from build123d import *

# Parameters (mm, degrees)
CROQUIS1_W                                           = 50
CROQUIS1_H                                           = 50
CROQUIS1_R                                           = 2
SALIENTE_EXTRUIR2_DEPTH                              = 100
CROQUIS4_W                                           = 3.2
CROQUIS4_H                                           = 40
SALIENTE_EXTRUIR5_DEPTH                              = 10.2
CROQUIS8_R                                           = 4
CORTAR_EXTRUIR3_DEPTH                                = 87.4
CORTAR_EXTRUIR2_START                                = -50
CROQUIS7_R                                           = 2
CORTAR_EXTRUIR2_DEPTH                                = 50
REFRENTADO_PARA_TORNILLO_TAP_N_CON_CABEZ_D           = 4.5
REFRENTADO_PARA_TORNILLO_TAP_N_CON_CABEZ_CSINK_D     = 8.96
REFRENTADO_PARA_TORNILLO_TAP_N_CON_CABEZ_CSINK_ANGLE = 90
SALIENTE_EXTRUIR6_DEPTH                              = 1.95
SALIENTE_EXTRUIR7_START                              = -4.5
SALIENTE_EXTRUIR7_DEPTH                              = 1.95
CORTAR_EXTRUIR4_DEPTH                                = 15.4


with BuildPart() as part:
    # Croquis1 → Saliente-Extruir2 (new body)
    with BuildSketch(Plane.XY):
        Rectangle(CROQUIS1_W, CROQUIS1_H)
        Circle(CROQUIS1_R, mode=Mode.SUBTRACT)
    extrude(amount=SALIENTE_EXTRUIR2_DEPTH)

    # Croquis2 → Cortar-Revolución1 (revolve, cut)
    with BuildSketch(Plane(origin=(0, 0, 0), x_dir=(0, 0, -1), z_dir=(1, 0, 0))):
        Polygon((-100, 15.2), (-100, 0), (-89.8, 0), (-89.8, 10), (-97.8, 15.2), align=None)
    revolve(axis=Axis((0, 0, 100), (0, 0, -1)), mode=Mode.SUBTRACT)

    # Croquis4 → Saliente-Extruir5 (add)
    with BuildSketch(Plane.XY.offset(100)):
        with Locations((-6.6, 0)):
            Rectangle(CROQUIS4_W, CROQUIS4_H)
        with Locations((6.6, 0)):
            Rectangle(CROQUIS4_W, CROQUIS4_H)
    extrude(amount=-SALIENTE_EXTRUIR5_DEPTH)

    # Croquis8 → Cortar-Extruir3 (cut)
    with BuildSketch(Plane.XY.offset(89.8)):
        Circle(CROQUIS8_R)
    extrude(amount=-CORTAR_EXTRUIR3_DEPTH, mode=Mode.SUBTRACT)

    # Croquis7 → Cortar-Extruir2 (cut)
    with BuildSketch(Plane.ZY.offset(25).offset(CORTAR_EXTRUIR2_START)):
        with Locations((95, 0)):
            Circle(CROQUIS7_R)
    extrude(amount=CORTAR_EXTRUIR2_DEPTH, mode=Mode.SUBTRACT)

    # Refrentado para tornillo tapón con cabeza plana de clavija de M41 (through all)
    with Locations(Plane.ZY.offset(25)):
        with Locations((95, 0)):
            CounterSinkHole(REFRENTADO_PARA_TORNILLO_TAP_N_CON_CABEZ_D / 2, REFRENTADO_PARA_TORNILLO_TAP_N_CON_CABEZ_CSINK_D / 2, counter_sink_angle=REFRENTADO_PARA_TORNILLO_TAP_N_CON_CABEZ_CSINK_ANGLE)

    # Croquis12 → Saliente-Extruir6 (add)
    with BuildSketch(Plane.ZY.offset(25)):
        Polygon((100, -25), (80, -25), (100, -45), align=None)
    extrude(amount=-SALIENTE_EXTRUIR6_DEPTH)

    # Croquis12<2> → Saliente-Extruir7 (add)
    with BuildSketch(Plane.ZY.offset(25).offset(SALIENTE_EXTRUIR7_START)):
        Polygon((100, -25), (80, -25), (100, -45), align=None)
    extrude(amount=-SALIENTE_EXTRUIR7_DEPTH)

    # Croquis13 → Cortar-Extruir4 (cut)
    with BuildSketch(Plane.XY.offset(100)):
        with BuildLine():
            Line((25, 25), (25, 14))
            Line((25, 14), (19, 14))
            ThreePointArc((19, 14), (15.464466094, 15.464466094), (14, 19))
            Line((14, 19), (14, 25))
            Line((14, 25), (25, 25))
        make_face()
    extrude(amount=-CORTAR_EXTRUIR4_DEPTH, mode=Mode.SUBTRACT)


solid = part.part
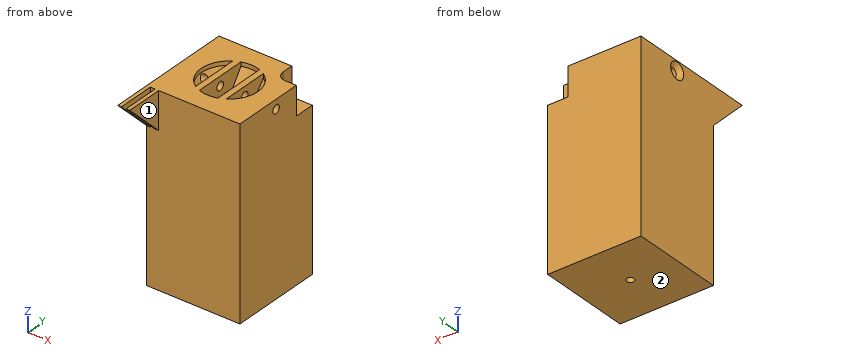
The listing builds one solid part. Answer for the finished solid, in the listing's coordinates (mm). Face numbers are marked on the shaded views. A direction names the side the tool comes from. Coordinates: 2 decimals unless noted, no trailing zeros. Write each loop counter-clockwise with the first axis right and the second up, starting at its lowest first coordinate (ties: lowest second). Pieces come first, ordered by that corner, then holes. Notation, with made-up numbers: (41.5, 88) - (82.5, 88) arc R16 ccw to (82.5, 93) - close; hole circle Ø7 at (86.25, 51.5). An arc over 180 degrees is marked (long way). Put each result on its own line as item: value.
1. The part is cut by section C-C on y = 0. State how many separate pieces and enclosed holes the cut face has, plus the area to 3 significant figures.
Answer sheet:
separate pieces: 6
enclosed holes: 0
area: 3,950 mm^2
2. Flat-ended cylindrical pins translate along their axes: pin 1 Ø2.5 at (x, y) = (0, 0) entering from +Z; pin 2 Ø0.5 at (x, y) = (9.5, -1.5) entering from +Z; pin 3 Ø10 at (y, z) = (-39, 92) entering from +X; pin 4 Ø10 at (x, z) = (4, 49) entering from -Y. Find the tip coordinate at first contact, or state that the pin passes through.
Answer sheet:
pin 1: passes through
pin 2: stops at z = 89.8
pin 3: stops at x = -18.55
pin 4: stops at y = -25
3. The part is cut by section B-B on z = 23.5. Give the vertices of the cut face in (x, y), plus the area to 3 significant figures.
Answer sheet:
outline: (-25, -25) - (25, -25) - (25, 25) - (-25, 25) - close; hole circle Ø8 at (0, 0)
area: 2,450 mm^2
4. The part is cut by section A-A on x = 0. Give the vertices of the cut face in (y, z), plus the area to 3 significant figures.
Answer sheet:
outline: (-25, 0) - (-2, 0) - (-2, 2.4) - (-4, 2.4) - (-4, 89.8) - (-10, 89.8) - (-15.2, 97.8) - (-15.2, 100) - (-25, 100) - close; (2, 0) - (25, 0) - (25, 100) - (15.2, 100) - (15.2, 97.8) - (10, 89.8) - (4, 89.8) - (4, 2.4) - (2, 2.4) - close
area: 4,020 mm^2
5. Find the intervals of material crossed by line 1 along Y through (x, z) = (-6.8, 95); line 2 along X through (y, z) = (0, 0.7); line 3 along Y through (x, z) = (0, 23), in increasing order. Write a range as from..to.
Answer sheet:
line 1: y = -25..-2.25, 2.25..25
line 2: x = -25..-2, 2..25
line 3: y = -25..-4, 4..25
6. A tool of negligible diameter and unlimited length cuts with its end or side. For the marked faces 1 and 2, from which of +Z, -Z, +X, -X, +Y, -Y can it reach the whole face along a straight path? Write none if from no direction.
Answer sheet:
face 1: +Z, -Z, +X, -Y
face 2: -Z, +X, -X, +Y, -Y
